Part print with two shaded views. Sizes in mm from the minimum x, y, z corner. Round coordinates to 2 decimals unless told otherwise and drop trailing zeros. Order: outer loops, then holes, each group sorted by start corner. A loop starts at its lowest first (then second) coordinate and runs counter-clockwise, first axis right, second up. Notation, with made-up numbers: (23.25, -19) -> (76.25, -19) arc R21 cw to (76.25, 20) -> close; hole circle Ø11 at (46.25, 53). An arc over 180 degrees is marked (long way). Answer as a JSON object with one key per item and string values.
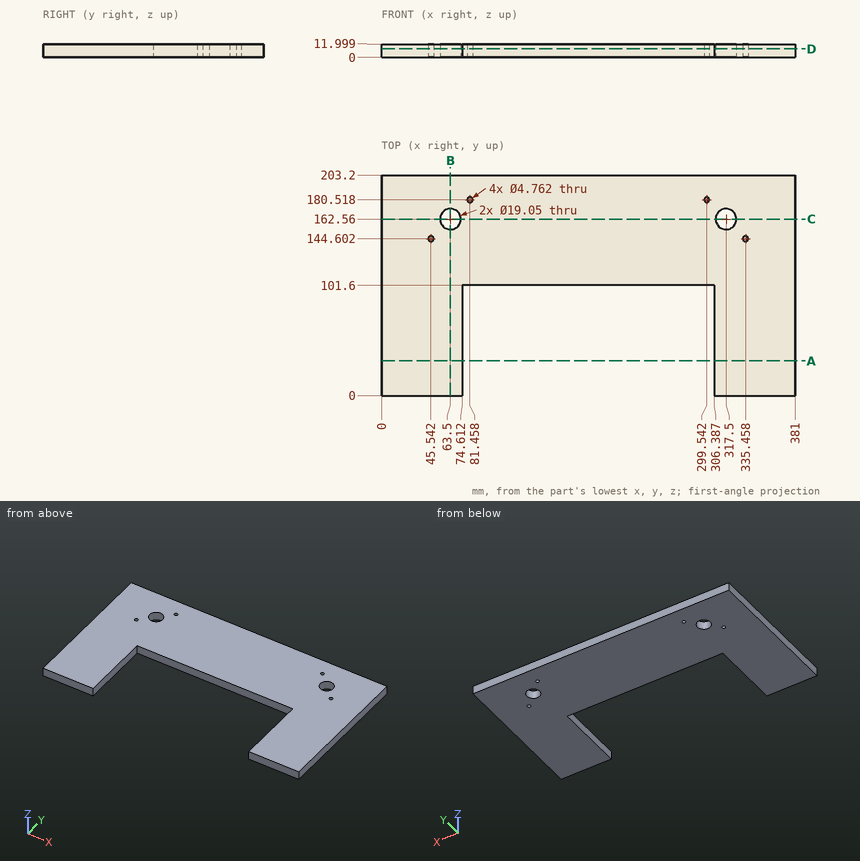
1) Cut at B-B, the plane x = 63.5. Give the cut face in (y, z) (1 decimal).
Checked values:
{"outline": "(0, 0) -> (153, 0) -> (153, 12) -> (0, 12) -> close; (172.1, 0) -> (203.2, 0) -> (203.2, 12) -> (172.1, 12) -> close"}
2) Flat gauge pins, fed straight in: pin 1 Ø4.5 at (x, y) = (45.54, 144.6) entering from -Z; pin 2 Ø6 at (x, z) = (163, 7.5) entering from -Y. Where does each tip first touch, or does it go through?
Checked values:
{"pin 1": "passes through", "pin 2": "stops at y = 101.6"}
3) Cut at D-D, the plane z = 7.5. Count the separate pieces of the cut face and the enclosed holes in it, plus the area to 3 significant figures.
Checked values:
{"separate pieces": "1", "enclosed holes": "6", "area": "53,200 mm²"}
4) Probe L1, parallel to X at y = 13.5, z = 4.25; L2, parallel to Y at x = 317.5, z = 6.25 (1 decimal); L3, parallel to X at y = 165.5, z = 6.5. List the from-to ranges inside material, lowest first. Write a range as from..to.
Checked values:
{"L1": "x = 0..74.61, 306.39..381", "L2": "y = 0..153, 172.1..203.2", "L3": "x = 0..54.44, 72.56..308.44, 326.56..381"}
5) Cut at C-C, the plane y = 162.56. Give the cut face in (x, z) (1 decimal).
Checked values:
{"outline": "(0, 0) -> (54, 0) -> (54, 12) -> (0, 12) -> close; (73, 0) -> (308, 0) -> (308, 12) -> (73, 12) -> close; (327, 0) -> (381, 0) -> (381, 12) -> (327, 12) -> close"}
6) Cut at A-A, the plane y = 32. Give the cut face in (x, z), plus the area to 3 significant figures.
Checked values:
{"outline": "(0, 0) -> (74.61, 0) -> (74.61, 12) -> (0, 12) -> close; (306.39, 0) -> (381, 0) -> (381, 12) -> (306.39, 12) -> close", "area": "1,790 mm²"}
